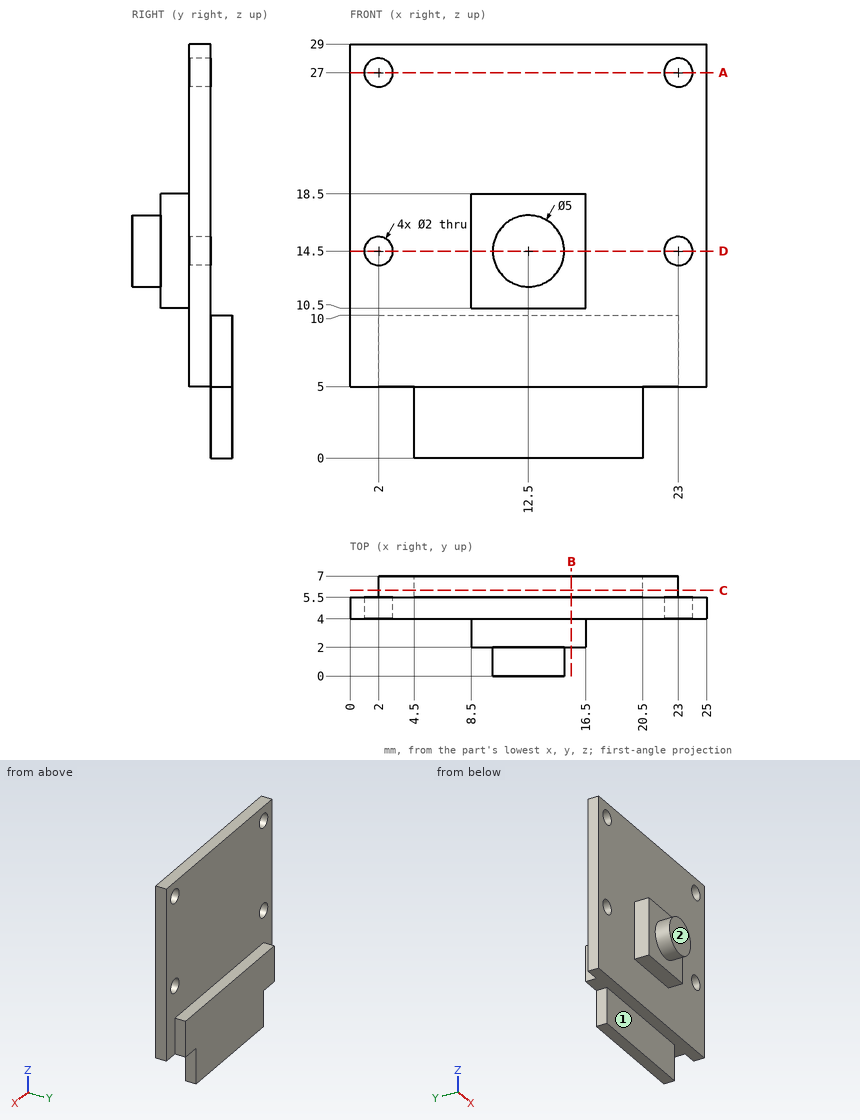
Print and shaded views of the part. All mm, measured from the part's lowest x, y and z. A direction names the side the tool comes from. Coordinates: 2 decimals unless noted, no trailing zeros. Order: outer loops, then holes, each group sorted by start corner. A loop starts at its lowest first (then second) coordinate and runs counter-clockwise, first axis right, second up. Notation, with made-up numbers: M 52.5,44.5 L 64.5,44.5 A18 cw 64.5,61.5 Z; hole C 49,43 d11. An arc over 180 degrees is marked long. Write each question's results on one line, items separated by ' | '. Start each with the question number.
Q1. Flat gauge pins, fed straight in: P1, Ø1.2, axis at y = 6.5, z = 1.5, coming from the +X side; P2, Ø2, axis at x = 13.5, y = 3.5, coming from the -Z side; P3, Ø4, axis at x = 10.5, z = 2.5, coming from the -Y side; P4, Ø1.6, axis at x = 2, z = 14.5, coming from the -Y side. Where does each tip first touch, or does it go through?
Q2. Which spindle directions (+Z, -Z, +X, -X, +Y, -Y) get a long thin tool onto all of the face, cutting with end or side? Do the marked faces 1 and 2. Say none if no direction does.
Q3. Cut at C-C (y = 6). List the corners of the cut face in (x, z), then the cut area to 3 significant figures.
Q4. Drill centre lines: probe 1 along Z at (x, y) = (2, 4.7); probe 2 along Y at (x, z) = (18.5, 7); probe 3 along Y at (x, z) = (12.75, 11.5). Where is each one in solid material? Low to high. Write a range as from..to.
Q5. Cut at A-A (z = 27). List the corners of the cut face in (x, y), then the cut area to 3 significant figures.
Q6. Cut at D-D (z = 14.5). List the corners of the cut face in (x, y), then the cut area to 3 significant figures.
Q7. Cut at B-B (x = 15.5). List the corners of the cut face in (y, z).
Found:
1) P1: x = 20.5 | P2: z = 5 | P3: y = 5.5 | P4: through
2) face 1: -Z, +X, -X, -Y | face 2: +Z, -Z, +X, -X, -Y
3) outline: M 2,5 L 4.5,5 L 4.5,0 L 20.5,0 L 20.5,5 L 23,5 L 23,10 L 2,10 Z | area: 185 mm²
4) probe 1: 5..13.5, 15.5..26, 28..29 | probe 2: 4..7 | probe 3: 2..5.5
5) outline: M 0,4 L 1,4 L 1,5.5 L 0,5.5 Z; M 3,4 L 22,4 L 22,5.5 L 3,5.5 Z; M 24,4 L 25,4 L 25,5.5 L 24,5.5 Z | area: 31.5 mm²
6) outline: M 0,4 L 1,4 L 1,5.5 L 0,5.5 Z; M 3,4 L 8.5,4 L 8.5,2 L 10,2 L 10,0 L 15,0 L 15,2 L 16.5,2 L 16.5,4 L 22,4 L 22,5.5 L 3,5.5 Z; M 24,4 L 25,4 L 25,5.5 L 24,5.5 Z | area: 57.5 mm²
7) outline: M 2,10.5 L 4,10.5 L 4,5 L 5.5,5 L 5.5,0 L 7,0 L 7,10 L 5.5,10 L 5.5,29 L 4,29 L 4,18.5 L 2,18.5 Z
